```python
from build123d import *

# Parameters (mm, degrees)
F0_R     = 2.5
F1_DEPTH = 3
F2_START = -2.5
F0_R_2   = 3.25
F2_DEPTH = 0.5
F3_DEPTH = 0.5
F4_SIZE2 = 0.74999
F4_SIZE  = 0.49999
F5_SIZE2 = 0.49999
F5_SIZE  = 0.74999


# Not quite as in the source:
# - a fillet or chamfer is up to 0.001 mm smaller than in the source, because OpenCascade refuses the exact size


with BuildPart() as f1:
    # F0 (on Top) → F1 (new body)
    with BuildSketch(Plane.XY):
        Circle(F0_R)
    extrude(amount=-F1_DEPTH)

    # F0 (on Top) → F2 (join)
    with BuildSketch(Plane.XY.offset(F2_START)):
        Circle(F0_R_2)
        Circle(F0_R, mode=Mode.SUBTRACT)
    extrude(amount=-F2_DEPTH)

    # F0 (on Top) → F3 (join)
    with BuildSketch(Plane.XY):
        Circle(F0_R_2)
        Circle(F0_R, mode=Mode.SUBTRACT)
    extrude(amount=-F3_DEPTH)

    # F4 (size 0.5 and 0.75 in the source; OpenCascade refuses exactly that, so slightly less here)
    f4_edges = [f1.edges().sort_by_distance(p)[0] for p in [
        (-3.25, 0, -0.5),
    ]]
    f4_side = f1.faces().sort_by_distance((-3.25, 0, -0.25))[0]
    chamfer(f4_edges, length=F4_SIZE, length2=F4_SIZE2, reference=f4_side)

    # F5 (size 0.75 and 0.5 in the source; OpenCascade refuses exactly that, so slightly less here)
    f5_edges = [f1.edges().sort_by_distance(p)[0] for p in [
        (-3.25, 0, -2.5),
    ]]
    f5_side = f1.faces().sort_by_distance((-3.158076, 0, -2.5))[0]
    chamfer(f5_edges, length=F5_SIZE, length2=F5_SIZE2, reference=f5_side)


solid = f1.part
```
CAD build for the part. Positions are in the model's coordinates, mm. Coordinates: 2 decimals unless noted, no trailing zeros. Loops run counter-clockwise (first coordinate to the right, second up) from the corner with the lowest first, then second, coordinate; pieces in that order, holes last. Notation, with made-up numbers: (58, 54.25) - (117, 54.25) arc R9 cw to (117, 62.25) - close; hole circle Ø2 at (45.25, 69). An arc over 180 degrees is marked (long way). Use CSV: the item, a comma, the result in double quotes. Start each with the question number.
Q1. Two-plate mould, pull along Z, no slides. Class faces 1 (the cylindrical face through (-0.54, -2.44, -1.49)), 2 (the flat face through (0, 0, -3)), 3 (the flat face through (0, 0, 0)): +Z half, -Z half, draft (parallel to the pull), parting line (faces both ways), or undercut.
Q2. Probe probe 1 along Z at (x, y) = (-1.5, -2.5); probe 2 along Z at (x, y) = (1.75, 2.25); probe 3 along X at (y, z) = (-2.25, -2.3). List the from-to ranges inside material, lowest first. Write a range as from..to.
Q3. Cut at C-C, the plane z = -0.95. List the corners of the cut face in (x, y).
Q4. Cut at D-D, the plane z = -0.2. List the corners of the cut face in (x, y), then the cut area to 3 significant figures.
Here are the results:
1,face 1,"undercut"
1,face 2,"-Z half"
1,face 3,"+Z half"
2,probe 1,"-3..-2.78, -0.22..0"
2,probe 2,"-3..-2.73, -0.27..0"
2,probe 3,"-1.09..1.09"
3,outline,"circle Ø5 at (0, 0)"
4,outline,"circle Ø5.9 at (0, 0)"
4,area,"27.3 mm2"
